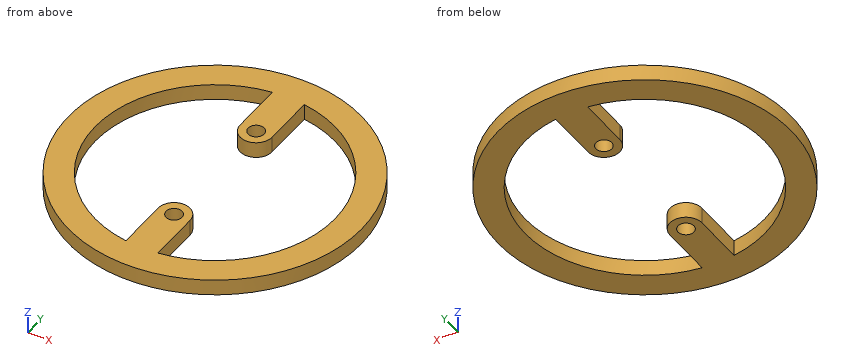
Autodesk Inventor part; units mm, degrees
ref_plane "YZ Plane" through (0, 0, 0) normal (1, 0, 0) x (0, 1, 0)
ref_plane "XZ Plane" through (0, 0, 0) normal (0, 1, 0) x (-1, 0, 0)
ref_plane "XY Plane" through (0, 0, 0) normal (0, 0, 1) x (1, 0, 0)
sketch "Sketch1" plane through (0, 0, 0) normal (0, 0, 1) x (1, 0, 0)
  circle A0 centre (0, 0) radius 27.5
  dimension "d0" = 55
extrude "Extrusion1" add sketch "Sketch1" along normal blind 3
sketch "Sketch2" plane through (0, 0, 3) normal (0, 0, 1) x (1, 0, 0)
  circle A0 centre (0, 0) radius 27.5
  circle A1 centre (0, 0) radius 22.5
  dimension "d3" = 45
extrude "Extrusion2" cut sketch "Sketch2" against normal up to next contours A1
sketch "Sketch4" plane through (0, 0, 3) normal (0, 0, 1) x (1, 0, 0)
  circle A0 centre (0, 0) radius 22.5
  line L0 (0, 12.5) -> (0, 22.5) construction
  line L1 (-3, 12.5) -> (-3, 22.5)
  line L2 (3, 22.5) -> (3, 12.5)
  arc A1 (-3, 12.5) -> (3, 12.5) centre (0, 12.5) ccw
  arc A2 (3, 22.5) -> (-3, 22.5) centre (0, 22.5) ccw
  point P0 (0, 17.5)
  dimension "d10" = 10
  dimension "d11" = 6
extrude "Extrusion4" add sketch "Sketch4" against normal up to surface (3 mm away) contours L2 A1 L1 A0 | A0 L1 A2 L2 picked at (-0.3342, 15.8259)
hole "Hole1" at (0, 12.5, 3) direction (0, 0, -1) diameter 3 end through all
mirror "Mirror1" about plane through (0, 0, 0) normal (0, 1, 0) of "Extrusion4", "Hole1"
properties part number "TreeHolder"
Work out the finished part from the listing and answer in its coordinate system (mm). Coordinates: 2 decimals unless noted, no trailing zeros. Write each loop counter-clockwise with the first axis right and the second up, starting at its lowest first coordinate (ties: lowest second). Pieces come first, ordered by that corner, then holes. Notation, with made-up numbers: M -20,85.5 L 36,85.5 A28 cw 36,108.5 Z; hole C 81,-34 d10. An arc over 180 degrees is marked long. Use one line per item in the form item = value. Start each with the question number.
1. The part is cut by section C-C (x = 16.5). Give the vertices of the cut face in (y, z), plus the area to 3 significant figures.
2. The part is cut by section B-B (x = 0). Give the vertices of the cut face in (y, z).
3. Each of these flat-tipped pins is pushed along its axis until it touches: P1, Ø0.9, axis at y = 19, z = 1, coming from the +X side; P2, Ø0.9, axis at y = -16, z = 1.5, coming from the +X side; P3, Ø0.9, axis at y = -18.5, z = 1, coming from the -X side; P4, Ø1, axis at y = -0.5, z = 0.5, coming from the +X side. Where does it stop, or does it pass through?
4. The part is cut by section D-D (y = 16). Give the vertices of the cut face in (x, z).
5. Straight lines are drawn through the part: probe 1 along Y at (x, z) = (0, 1.4); probe 2 along X at (y, z) = (-18.5, 2.8); probe 3 along Y at (x, z) = (0.5, 0.25). For each, find the intervals that lie inside material, in ascending order. Write a range as from..to.
6. The part is cut by section A-A (y = 0). Give the vertices of the cut face in (x, z), plus the area to 3 significant figures.
Evaluation:
q1.outline = M -22,0 L -15.3,0 L -15.3,3 L -22,3 Z; M 15.3,0 L 22,0 L 22,3 L 15.3,3 Z
q1.area = 40.2 mm^2
q2.outline = M -27.5,0 L -14,0 L -14,3 L -27.5,3 Z; M -11,0 L -9.5,0 L -9.5,3 L -11,3 Z; M 9.5,0 L 11,0 L 11,3 L 9.5,3 Z; M 14,0 L 27.5,0 L 27.5,3 L 14,3 Z
q3.P1 = 20.3
q3.P2 = 22.68
q3.P3 = -20.75
q3.P4 = 27.5
q4.outline = M -22.37,0 L -15.82,0 L -15.82,3 L -22.37,3 Z; M -3,0 L 3,0 L 3,3 L -3,3 Z; M 15.82,0 L 22.37,0 L 22.37,3 L 15.82,3 Z
q5.probe_1 = -27.5..-14, -11..-9.5, 9.5..11, 14..27.5
q5.probe_2 = -20.35..-12.81, -3..3, 12.81..20.35
q5.probe_3 = -27.5..-13.91, -11.09..-9.54, 9.54..11.09, 13.91..27.5
q6.outline = M -27.5,0 L -22.5,0 L -22.5,3 L -27.5,3 Z; M 22.5,0 L 27.5,0 L 27.5,3 L 22.5,3 Z
q6.area = 30.0 mm^2
